Source: three-view drawing plus pictorial views. Frame: mm from the lowest corner of the part. Give positions to 0.01 mm unless a question says otherwise; leave off trailing zeros. Order: outer loops, then holes, each group sorted by start corner. A loop starts at its lowest first (then second) coordinate and runs counter-clockwise, first axis right, second up. Notation, with made-up numbers: (36.25, 77) -> (63.25, 77) arc R14 ccw to (63.25, 93) -> close; hole circle Ø10 at (31, 66.25). An arc over 180 degrees is marked (long way). Answer in a Markdown table with one row per item.
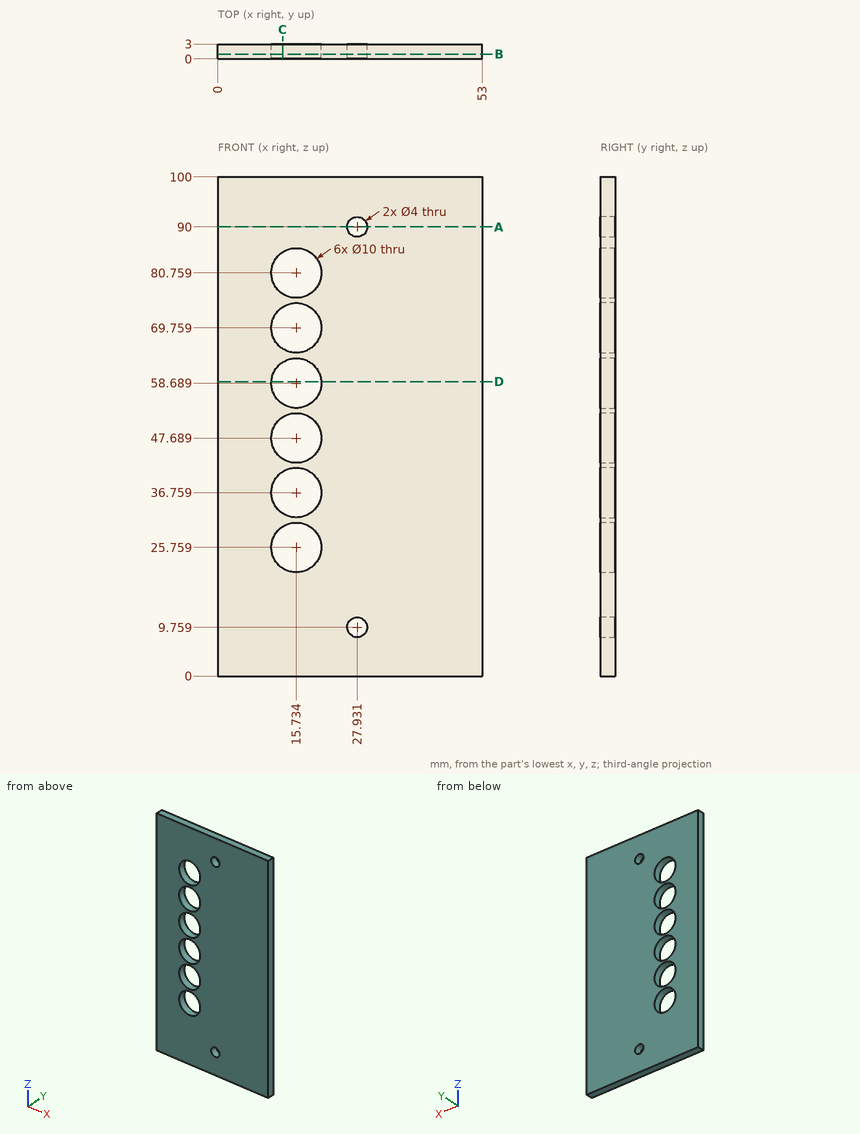
(1) Section query C-C (x = 13). Return the cut outline in (y, z) (1 decimal), plus the area to 3 significant figures.
A:
| item | result |
|---|---|
| outline | (0, 0) -> (3, 0) -> (3, 21.6) -> (0, 21.6) -> close; (0, 29.9) -> (3, 29.9) -> (3, 32.6) -> (0, 32.6) -> close; (0, 40.9) -> (3, 40.9) -> (3, 43.5) -> (0, 43.5) -> close; (0, 51.9) -> (3, 51.9) -> (3, 54.5) -> (0, 54.5) -> close; (0, 62.9) -> (3, 62.9) -> (3, 65.6) -> (0, 65.6) -> close; (0, 73.9) -> (3, 73.9) -> (3, 76.6) -> (0, 76.6) -> close; (0, 84.9) -> (3, 84.9) -> (3, 100) -> (0, 100) -> close |
| area | 149 mm^2 |
(2) Section query A-A (z = 90). Return the cut outline in (x, y).
A:
| item | result |
|---|---|
| outline | (0, 0) -> (25.93, 0) -> (25.93, 3) -> (0, 3) -> close; (29.93, 0) -> (53, 0) -> (53, 3) -> (29.93, 3) -> close |
(3) Section query B-B (y = 0.95). Give the number of separate pieces and of enclosed holes in the cut face, plus the area to 3 significant figures.
A:
| item | result |
|---|---|
| separate pieces | 1 |
| enclosed holes | 8 |
| area | 4,800 mm^2 |
(4) Section query D-D (z = 59). Return the cut outline in (x, y).
A:
| item | result |
|---|---|
| outline | (0, 0) -> (10.74, 0) -> (10.74, 3) -> (0, 3) -> close; (20.72, 0) -> (53, 0) -> (53, 3) -> (20.72, 3) -> close |
(5) First-contact query: pin 1 Ø6 at (x, z) = (15.73, 80.76) entering from -Y. Flat tip, straight axial feed; report the tip coordinate or a pass-through.
A:
| item | result |
|---|---|
| pin 1 | passes through |
(6) Ray query, probe 1 along X at (y, z) = (1.45, 90); probe 2 along X at (y, z) = (0.95, 26). Return the intervals inside material, ascending.
A:
| item | result |
|---|---|
| probe 1 | x = 0 to 25.93, 29.93 to 53 |
| probe 2 | x = 0 to 10.74, 20.73 to 53 |
